```python
from build123d import *

# Parameters (mm, degrees)
ESBO_O1_W                  = 60
ESBO_O1_H                  = 110
ESBO_O1_R                  = 25
RESSALTO_EXTRUS_O1_DEPTH   = 2
ESBO_O2_W                  = 110
ESBO_O2_H                  = 77
RESSALTO_EXTRUS_O2_DEPTH   = 2
ESBO_O5_R                  = 13.5
ESBO_O5_R_2                = 1
CORTE_EXTRUS_O3_DEPTH      = 10
ESBO_O6_R                  = 2.5
CORTE_EXTRUS_O4_DEPTH      = 10
ESBO_O8_R                  = 5
CORTE_EXTRUS_O7_DEPTH      = 115.236596588
CORTE_EXTRUS_O7_DEPTH_BACK = 115.236596588
ESBO_O9_R                  = 2.5
CORTE_EXTRUS_O8_DEPTH      = 10
ESBO_O12_R                 = 2.5
CORTE_EXTRUS_O9_DEPTH      = 10
CORTE_EXTRUS_O10_REACH     = 116.237
ESBO_O13_R                 = 2.5
ESBO_O15_R                 = 3.5
CORTE_EXTRUS_O11_DEPTH     = 10
CUT_EXTRUDE1_REACH         = 116.237
SKETCH1_R                  = 2.5


with BuildPart() as part:
    # Esboço1 → Ressalto-extrusão1 (new body)
    with BuildSketch(Plane(origin=(0, 0, 0), x_dir=(1, 0, 0), z_dir=(0, 1, 0))):
        Rectangle(ESBO_O1_W, ESBO_O1_H)
        Circle(ESBO_O1_R, mode=Mode.SUBTRACT)
        Circle(ESBO_O1_R)
    extrude(amount=RESSALTO_EXTRUS_O1_DEPTH)

    # Esboço2 → Ressalto-extrusão2 (add)
    with BuildSketch(Plane.ZY.offset(30)):
        with Locations((0, 38.5)):
            Rectangle(ESBO_O2_W, ESBO_O2_H)
    ressalto_extrus_o2 = extrude(amount=RESSALTO_EXTRUS_O2_DEPTH)

    # Espelhar1: Ressalto-extrusão2 across plane
    add(ressalto_extrus_o2.mirror(Plane(origin=(0, 0, 0), x_dir=(0, 0, 1), z_dir=(1, 0, 0))))

    # Esboço5 → Corte-extrusão3 (cut)
    with BuildSketch(Plane(origin=(-30, 0, 0), x_dir=(0, 0, -1), z_dir=(1, 0, 0))):
        with Locations((0, 20.625)):
            Circle(ESBO_O5_R)
        with Locations((0, 20.625)):
            Circle(ESBO_O5_R_2, mode=Mode.SUBTRACT)
        with Locations((0, 20.625)):
            Circle(ESBO_O5_R_2)
    extrude(amount=-CORTE_EXTRUS_O3_DEPTH, mode=Mode.SUBTRACT)

    # Esboço6 → Corte-extrusão4 (cut)
    with BuildSketch(Plane.ZY.offset(32)):
        with Locations((45, 20.625)):
            Circle(ESBO_O6_R)
        with Locations((-6, 65.225)):
            Circle(ESBO_O6_R)
        with Locations((-43.5, 31.925)):
            Circle(ESBO_O6_R)
    extrude(amount=-CORTE_EXTRUS_O4_DEPTH, mode=Mode.SUBTRACT)

    # Esboço8 → Corte-extrusão7 (cut, two sides)
    with BuildSketch(Plane.ZY.offset(32)) as corte_extrus_o7_sk:
        with Locations((0, 45.125)):
            Circle(ESBO_O8_R)
    extrude(amount=CORTE_EXTRUS_O7_DEPTH, mode=Mode.SUBTRACT)
    extrude(corte_extrus_o7_sk.sketch, amount=-CORTE_EXTRUS_O7_DEPTH_BACK, mode=Mode.SUBTRACT)

    # Esboço9 → Corte-extrusão8 (cut)
    with BuildSketch(Plane(origin=(0, 2, 0), x_dir=(1, 0, 0), z_dir=(0, 1, 0))):
        with Locations(Location((-8.838834765, 8.838834765, 0), (0, 0, 270))):
            Circle(ESBO_O9_R)
        with Locations(Location((-8.838834765, -8.838834765, 0), (0, 0, 270))):
            Circle(ESBO_O9_R)
        with Locations(Location((8.838834765, 8.838834765, 0), (0, 0, 270))):
            Circle(ESBO_O9_R)
        with Locations(Location((8.838834765, -8.838834765, 0), (0, 0, 270))):
            Circle(ESBO_O9_R)
    extrude(amount=-CORTE_EXTRUS_O8_DEPTH, mode=Mode.SUBTRACT)

    # Esboço12 → Corte-extrusão9 (cut)
    with BuildSketch(Plane(origin=(32, 0, 0), x_dir=(0, 0, -1), z_dir=(1, 0, 0))):
        with Locations((45.5, 31.925)):
            Circle(ESBO_O12_R)
        with Locations((-45.5, 20.625)):
            Circle(ESBO_O12_R)
    extrude(amount=-CORTE_EXTRUS_O9_DEPTH, mode=Mode.SUBTRACT)

    # Esboço13 → Corte-extrusão10 (cut, up to next)
    with BuildSketch(Plane.ZY.offset(32), mode=Mode.PRIVATE) as corte_extrus_o10_sk1:
        with Locations((-44.5, 67)):
            Circle(ESBO_O13_R)
    corte_extrus_o10_tool1 = extrude(corte_extrus_o10_sk1.sketch, amount=-CORTE_EXTRUS_O10_REACH, mode=Mode.PRIVATE) & part.part
    # Esboço13 → Corte-extrusão10 (cut, up to next)
    with BuildSketch(Plane.ZY.offset(32), mode=Mode.PRIVATE) as corte_extrus_o10_sk2:
        with Locations(Location((44.5, 67, 0), (0, 0, 180))):
            Circle(ESBO_O13_R)
    corte_extrus_o10_tool2 = extrude(corte_extrus_o10_sk2.sketch, amount=-CORTE_EXTRUS_O10_REACH, mode=Mode.PRIVATE) & part.part
    add(corte_extrus_o10_tool1.solids().sort_by_distance((-32, 67, -44.5))[0], mode=Mode.SUBTRACT)
    add(corte_extrus_o10_tool2.solids().sort_by_distance((-32, 67, 44.5))[0], mode=Mode.SUBTRACT)

    # Esboço15 → Corte-extrusão11 (cut)
    with BuildSketch(Plane(origin=(32, 0, 0), x_dir=(0, 0, -1), z_dir=(1, 0, 0))):
        with Locations((-22.5, 45.125)):
            Circle(ESBO_O15_R)
        with Locations((22.5, 45.125)):
            Circle(ESBO_O15_R)
    extrude(amount=-CORTE_EXTRUS_O11_DEPTH, mode=Mode.SUBTRACT)

    # Sketch1 → Cut-Extrude1 (cut, up to next)
    with BuildSketch(Plane(origin=(32, 0, 0), x_dir=(0, 0, -1), z_dir=(1, 0, 0)), mode=Mode.PRIVATE) as cut_extrude1_sk1:
        with Locations((45.5, 67)):
            Circle(SKETCH1_R)
    cut_extrude1_tool1 = extrude(cut_extrude1_sk1.sketch, amount=-CUT_EXTRUDE1_REACH, mode=Mode.PRIVATE) & part.part
    # Sketch1 → Cut-Extrude1 (cut, up to next)
    with BuildSketch(Plane(origin=(32, 0, 0), x_dir=(0, 0, -1), z_dir=(1, 0, 0)), mode=Mode.PRIVATE) as cut_extrude1_sk2:
        with Locations(Location((-45.5, 67, 0), (0, 0, 180))):
            Circle(SKETCH1_R)
    cut_extrude1_tool2 = extrude(cut_extrude1_sk2.sketch, amount=-CUT_EXTRUDE1_REACH, mode=Mode.PRIVATE) & part.part
    add(cut_extrude1_tool1.solids().sort_by_distance((32, 67, -45.5))[0], mode=Mode.SUBTRACT)
    add(cut_extrude1_tool2.solids().sort_by_distance((32, 67, 45.5))[0], mode=Mode.SUBTRACT)


solid = part.part
```
Check sheet for the modelled part. Datum: model origin and axes. Units: mm. A direction names the side the tool comes from. Round coordinates to 2 decimals unless told otherwise and drop trailing zeros. Loops run counter-clockwise (first coordinate to the right, second up) from the corner with the lowest first, then second, coordinate; pieces in that order, holes last. Notation, with made-up numbers: (-29, -16) -> (-7, -16) arc R17 ccw to (-7, 6) -> close; hole circle Ø7 at (56, 76.5). An arc over 180 degrees is marked (long way). Answer in a Markdown table with one row per item.
Q1. Sectioned sample at D-D on x = 23. Enter the section's corners in (y, z).
Data:
| item | result |
|---|---|
| outline | (0, -55) -> (2, -55) -> (2, 55) -> (0, 55) -> close |
Q2. Set-up check for faces 1 (the face through (31.014, 48.595, 22.956)), 2 (the face through (-11.28, 1.01, -9.38)), 3 (the face through (-30.986, 32.008, -7.258)), 4 (the face through (-30, 40, -1)), 5 (the face through (0, 1, 55)): record each of +Z, -Z, +X, -X, +Y, -Y from which the full face is reachable in a straight line by a thin tool's end or side.
Data:
| item | result |
|---|---|
| face 1 | +X |
| face 2 | +Y, -Y |
| face 3 | -X |
| face 4 | +Z, -Z, +Y |
| face 5 | +Z, +X, -X, +Y, -Y |
Q3. Release check for a two-part mould opening along Y. For faces 6 (the face through (-31.014, 67.704, -6.325)), 7 (the face through (0, 2, -1)), 8 (the face through (32, 39, -1)) record: released by +Y, released by -Y, zero draft, split by the parting line, or undercut.
Data:
| item | result |
|---|---|
| face 6 | undercut |
| face 7 | released by +Y |
| face 8 | zero draft |
Q4. Go/stop test with flat-tipped pins: P1, Ø8, axis at x = 8.84, z = -8.84, coming from the +Y side; P2, Ø4.5, axis at y = 31.925, z = -43.5, coming from the -X side. Record where each tip stops, or that it passes through.
Data:
| item | result |
|---|---|
| P1 | stops at y = 2 |
| P2 | stops at x = 30 |
Q5. Thickness scan on L1, parallel to Y at x = 31.55, z = -45.5 (3 decimals); L2, parallel to Y at x = -30.75, z = 0 (3 decimals); L3, parallel to X at y = 59.5, z = 7.5. Record the ranges inside material, lowest first.
Data:
| item | result |
|---|---|
| L1 | y = 0 to 29.425, 34.425 to 64.5, 69.5 to 77 |
| L2 | y = 0 to 7.125, 34.125 to 40.125, 50.125 to 77 |
| L3 | x = -32 to -30, 30 to 32 |
Q6. Sectioned sample at C-C on y = 10. Enter the section's corners in (x, z).
Data:
| item | result |
|---|---|
| outline | (-32, -55) -> (-30, -55) -> (-30, -8.33) -> (-32, -8.33) -> close; (-32, 8.33) -> (-30, 8.33) -> (-30, 55) -> (-32, 55) -> close; (30, -55) -> (32, -55) -> (32, 55) -> (30, 55) -> close |
Q7. Sectioned sample at A-A on z = 0. Enter the section's corners in (x, y) (3 decimals), then the cut area to 3 significant figures.
Data:
| item | result |
|---|---|
| outline | (-32, 0) -> (32, 0) -> (32, 40.125) -> (30, 40.125) -> (30, 2) -> (-30, 2) -> (-30, 7.125) -> (-32, 7.125) -> close; (-32, 34.125) -> (-30, 34.125) -> (-30, 40.125) -> (-32, 40.125) -> close; (-32, 50.125) -> (-30, 50.125) -> (-30, 77) -> (-32, 77) -> close; (30, 50.125) -> (32, 50.125) -> (32, 77) -> (30, 77) -> close |
| area | 334 mm^2 |
Q8. Sectioned sample at B-B on z = 44.5. Enter the section's corners in (x, y), then the cut area to 3 significant figures.
Data:
| item | result |
|---|---|
| outline | (-32, 0) -> (32, 0) -> (32, 18.33) -> (30, 18.33) -> (30, 2) -> (-30, 2) -> (-30, 18.18) -> (-32, 18.18) -> close; (-32, 23.07) -> (-30, 23.07) -> (-30, 64.5) -> (-32, 64.5) -> close; (-32, 69.5) -> (-30, 69.5) -> (-30, 77) -> (-32, 77) -> close; (30, 22.92) -> (32, 22.92) -> (32, 64.71) -> (30, 64.71) -> close; (30, 69.29) -> (32, 69.29) -> (32, 77) -> (30, 77) -> close |
| area | 390 mm^2 |
